Model file for the job. Use its own axes, mm. A direction names the side the tool comes from. Coordinates: 2 decimals unless noted, no trailing zeros. Write each loop counter-clockwise with the first axis right and the second up, starting at its lowest first coordinate (ties: lowest second). Pieces come first, ordered by that corner, then holes. Notation, with made-up numbers: (52.5, 16) -> (76.5, 16) arc R11 ccw to (76.5, 32) -> close; hole circle Ø10 at (-6.75, 9). An arc over 180 degrees is marked (long way). Answer as a JSON object with one key per item and string values. Group by question number.
from build123d import *

# Parameters (mm, degrees)
F1_DEPTH = 101.6
F2_W     = 25.4
F2_H     = 101.6
F3_DEPTH = 12.7
F5_DEPTH = 76.201


with BuildPart() as f1:
    # F0 (on Top) → F1 (new body)
    with BuildSketch(Plane.XY):
        Polygon((0, 76.2), (0, 0), (152.4, 76.2), align=None)
    extrude(amount=-F1_DEPTH)

    # F2 (on face) → F3 (cut)
    with BuildSketch(Plane(origin=(0, 76.2, 0), x_dir=(-1, 0, 0), z_dir=(0, 1, 0))):
        with Locations((-76.2, -50.8)):
            Rectangle(F2_W, F2_H)
    extrude(amount=-F3_DEPTH, mode=Mode.SUBTRACT)

    # F4 (on face) → F5 (cut, through all)
    with BuildSketch(Plane(origin=(0, 76.2, 0), x_dir=(-1, 0, 0), z_dir=(0, 1, 0))):
        with BuildLine():
            ThreePointArc((-88.9, -72.5728585247), (-63.5591417828, -72.4710526239), (-50.9180106878, -50.5081005394))
            ThreePointArc((-50.9180106878, -50.5081005394), (-63.5591417828, -28.545148455), (-88.9, -28.4433425542))
            Line((-88.9, -28.4433425542), (-88.9, -72.5728585247))
        make_face()
        with BuildLine():
            Line((-88.9, -72.5728585247), (-88.9, -28.4433425542))
            ThreePointArc((-88.9, -28.4433425542), (-101.7180106878, -50.5081005394), (-88.9, -72.5728585247))
        make_face()
    extrude(amount=-F5_DEPTH, mode=Mode.SUBTRACT)


solid = f1.part
(1) 3-axis set-ups, long thin cutter, end or side, ignore diameter. For faces 1 (the face through (76, 63.5, -14)), 2 (the face through (121, 76.2, -50)): which of +Z, -Z, +X, -X, +Y, -Y reach the whole face in a straight line?
(2) Pin check, flat tips, straight feed: pin 1 (4 mm diameter, centred on y = 70.5, z = -14, fed in from +X); pin 2 (4 mm diameter, centred on y = 72, z = -16, fed in from -X); pin 3 (6.5 mm diameter, centred on y = 68, z = -91, fed in from +X); pin 4 (8 mm diameter, centred on x = 29, z = -64.5, fed in from -Y). Stop position of each tip, or through.
(3) Cut at D-D on z = -92. List the corners of the cut face in (x, y), plus the area to 3 significant figures.
(4) Cut at A-A on z = -56. List the corners of the cut face in (x, y), plus the area to 3 significant figures.
(5) Cut at B-B on x = 70. List the corners of the cut face in (y, z).
(6) Wall check: probe 1 along X at (y, z) = (73.5, -10); probe 2 along Z at (x, y) = (84.5, 53); probe 3 along Z at (x, y) = (56.5, 51). Give the ranges that are in metal, low to high.
(7) Pull direction X, two halves, no side cores. Call faces 3 (the face through (88.9, 70, -14)), 4 (the face through (58, 47, -101.6)), 5 (the face through (63.5, 70, -14)), 6 (the face through (92, 46, -73)): released by +X, released by -X, zero draft, split by the parting line, or undercut.
(8) Cut at C-C on y = 53.5. List the corners of the cut face in (x, z).
Results found:
{
 "1": {"face 1": "+Z, -Z, +Y", "face 2": "+Z, -Z, +X, -X, +Y"},
 "2": {"pin 1": "stops at x = 145", "pin 2": "stops at x = 0", "pin 3": "stops at x = 142.5", "pin 4": "stops at y = 12.5"},
 "3": {"outline": "(0, 0) -> (152.4, 76.2) -> (88.9, 76.2) -> (88.9, 63.5) -> (63.5, 63.5) -> (63.5, 76.2) -> (0, 76.2) -> close", "area": "5,480 mm²"},
 "4": {"outline": "(0, 0) -> (51.52, 25.76) -> (51.52, 76.2) -> (0, 76.2) -> close; (101.12, 50.56) -> (152.4, 76.2) -> (101.12, 76.2) -> close", "area": "3,920 mm²"},
 "5": {"outline": "(35, -101.6) -> (63.5, -101.6) -> (63.5, -75.11) -> (35, -75.11) -> close; (35, -25.91) -> (63.5, -25.91) -> (63.5, 0) -> (35, 0) -> close"},
 "6": {"probe 1": "x = 0 to 63.5, 88.9 to 147", "probe 2": "z = -101.6 to -74.55, -26.46 to 0", "probe 3": "z = -101.6 to -66.4, -34.62 to 0"},
 "7": {"face 3": "undercut", "face 4": "zero draft", "face 5": "undercut", "face 6": "released by +X"},
 "8": {"outline": "(0, -101.6) -> (107, -101.6) -> (107, 0) -> (0, 0) -> close; hole circle Ø50.8 at (76.32, -50.51)"}
}
